Part model, mm, in its own coordinate system. Face numbers are marked on the shaded views. A direction names the side the tool comes from. Round coordinates to 2 decimals unless told otherwise and drop trailing zeros. Write each loop counter-clockwise with the first axis right and the second up, starting at its lowest first coordinate (ties: lowest second). Pieces come first, ordered by that corner, then holes. Notation, with made-up numbers: (-29.75, -17.75) -> (15.25, -17.75) arc R28 ccw to (15.25, 1.25) -> close; hole circle Ø5 at (43, 20.25). An arc over 180 degrees is marked (long way). Use CSV: the item, a comma, the result in double quotes. Start each with the question number.
(1) Saw through at D-D (x = 12). Give the cut face in (y, z), plus the area to 3 significant figures.
(2) Drop flat-ended pins along their axis: pin 1 (1.5 mm diameter, centred on x = -2.5, z = -1, fed in from -Y); pin 2 (1.5 mm diameter, centred on y = 2.5, z = -12, fed in from +X); pin 3 (0.6 mm diameter, centred on x = -3.5, y = 1.5, fed in from +Z). Give the stop position or say it passes through.
(3) Two-plate mould, pull along X, no slides. Class the marked faces 1, 2 and 3: released by +X, released by -X, zero draft, split by the parting line, or undercut.
(4) Saw through at C-C (y = 6.25). Give the cut face in (x, z), plus the area to 3 significant figures.
(5) Saw through at B-B (z = 20). Give the cut face in (x, y), plus the area to 3 significant figures.
(6) Which spindle directions (+Z, -Z, +X, -X, +Y, -Y) get a long thin tool onto all of the face, cutting with end or side? Do the marked faces 4 and 5. Say none if no direction does.
(7) Probe line 1 (Z direction, x = 0, y = 2.7); line 2 (Y direction, x = 5.5, z = -3.5). List the from-to ranges inside material, lowest first. Write a range as [from, to].
(8) Saw through at A-A (x = 0). Give the cut face in (y, z), plus the area to 4 significant figures.
```python
from build123d import *

# Parameters (mm, degrees)
CROQUIS1_R              = 23.5
SALIENTE_EXTRUIR1_DEPTH = 10
CORTAR_EXTRUIR3_DEPTH   = 5
CROQUIS3_R              = 1.25
CORTAR_EXTRUIR4_DEPTH   = 10
CORTAR_EXTRUIR6_DEPTH   = 2


with BuildPart() as part:
    # Croquis1 → Saliente-Extruir1 (new body)
    with BuildSketch(Plane(origin=(0, 0, 0), x_dir=(1, 0, 0), z_dir=(0, 1, 0))):
        Circle(CROQUIS1_R)
    extrude(amount=SALIENTE_EXTRUIR1_DEPTH)

    # Croquis2 → Cortar-Extruir3 (cut)
    with BuildSketch(Plane(origin=(0, 10, 0), x_dir=(1, 0, 0), z_dir=(0, 1, 0))):
        with BuildLine():
            ThreePointArc((3.5, 17), (0, 20.5), (-3.5, 17))
            Line((-3.5, 17), (3.5, 17))
        make_face()
        with BuildLine():
            Line((3.5, 17), (-3.5, 17))
            ThreePointArc((-3.5, 17), (0, 13.5), (3.5, 17))
        make_face()
        with BuildLine():
            Line((-3.5, 6.062177826), (-3.5, 17))
            Line((-3.5, 17), (-6.430705394, 2.765145228))
            ThreePointArc((-6.430705394, 2.765145228), (-5.231857547, 4.650555516), (-3.5, 6.062177826))
        make_face()
        with BuildLine():
            ThreePointArc((3.5, 17), (0, 13.5), (-3.5, 17))
            Line((-3.5, 17), (-3.5, 6.062177826))
            ThreePointArc((-3.5, 6.062177826), (0, 7), (3.5, 6.062177826))
            Line((3.5, 6.062177826), (3.5, 17))
        make_face()
        with BuildLine():
            Line((6.430705394, 2.765145228), (3.5, 17))
            Line((3.5, 17), (3.5, 6.062177826))
            ThreePointArc((3.5, 6.062177826), (5.231857547, 4.650555516), (6.430705394, 2.765145228))
        make_face()
        with BuildLine():
            ThreePointArc((6.430705394, 2.765145228), (5.231857547, 4.650555516), (3.5, 6.062177826))
            Line((3.5, 6.062177826), (3.5, 0))
            Line((3.5, 0), (7, 0))
            Line((7, 0), (6.430705394, 2.765145228))
        make_face()
        with BuildLine():
            ThreePointArc((3.5, 6.062177826), (0, 7), (-3.5, 6.062177826))
            Line((-3.5, 6.062177826), (-3.5, 0))
            Line((-3.5, 0), (3.5, 0))
            Line((3.5, 0), (3.5, 6.062177826))
        make_face()
        with BuildLine():
            Line((3.5, 0), (-3.5, 0))
            Line((-3.5, 0), (-3.5, -6.062177826))
            ThreePointArc((-3.5, -6.062177826), (0, -7), (3.5, -6.062177826))
            Line((3.5, -6.062177826), (3.5, 0))
        make_face()
        with BuildLine():
            ThreePointArc((-3.5, 6.062177826), (-5.231857547, 4.650555516), (-6.430705394, 2.765145228))
            Line((-6.430705394, 2.765145228), (-7, 0))
            Line((-7, 0), (-3.5, 0))
            Line((-3.5, 0), (-3.5, 6.062177826))
        make_face()
        with BuildLine():
            Line((-3.5, 0), (-7, 0))
            ThreePointArc((-7, 0), (-6.062177826, -3.5), (-3.5, -6.062177826))
            Line((-3.5, -6.062177826), (-3.5, 0))
        make_face()
        with BuildLine():
            Line((7, 0), (3.5, 0))
            Line((3.5, 0), (3.5, -6.062177826))
            ThreePointArc((3.5, -6.062177826), (6.062177826, -3.5), (7, 0))
        make_face()
        with BuildLine():
            ThreePointArc((7, 0), (6.856199303, 1.411570445), (6.430705394, 2.765145228))
            Line((6.430705394, 2.765145228), (7, 0))
        make_face()
        with BuildLine():
            Line((-7, 0), (-6.430705394, 2.765145228))
            ThreePointArc((-6.430705394, 2.765145228), (-6.856199303, 1.411570445), (-7, 0))
        make_face()
        with BuildLine():
            ThreePointArc((3.5, -6.062177826), (0, -7), (-3.5, -6.062177826))
            Line((-3.5, -6.062177826), (-3.5, -17))
            Line((-3.5, -17), (3.5, -17))
            Line((3.5, -17), (3.5, -6.062177826))
        make_face()
        with BuildLine():
            ThreePointArc((-3.5, -6.062177826), (-6.062177826, -3.5), (-7, 0))
            Line((-7, 0), (-7, -22.433234274))
            ThreePointArc((-7, -22.433234274), (-3.540409196, -23.231777864), (0, -23.5))
            ThreePointArc((0, -23.5), (3.540409196, -23.231777864), (7, -22.433234274))
            Line((7, -22.433234274), (7, 0))
            ThreePointArc((7, 0), (6.062177826, -3.5), (3.5, -6.062177826))
            Line((3.5, -6.062177826), (3.5, -17))
            Line((3.5, -17), (-3.5, -17))
            Line((-3.5, -17), (-3.5, -6.062177826))
        make_face()
    extrude(amount=-CORTAR_EXTRUIR3_DEPTH, mode=Mode.SUBTRACT)

    # Croquis3 → Cortar-Extruir4 (cut)
    with BuildSketch(Plane(origin=(0, 10, 0), x_dir=(1, 0, 0), z_dir=(0, 1, 0))):
        Circle(CROQUIS3_R)
    extrude(amount=-CORTAR_EXTRUIR4_DEPTH, mode=Mode.SUBTRACT)

    # Croquis5 → Cortar-Extruir6 (cut)
    with BuildSketch(Plane.XZ):
        with BuildLine():
            Line((-7.5, 2.5), (7.5, 2.5))
            ThreePointArc((7.5, 2.5), (10, 0), (7.5, -2.5))
            Line((7.5, -2.5), (-7.5, -2.5))
            ThreePointArc((-7.5, -2.5), (-10, 0), (-7.5, 2.5))
        make_face()
    extrude(amount=-CORTAR_EXTRUIR6_DEPTH, mode=Mode.SUBTRACT)


solid = part.part
```
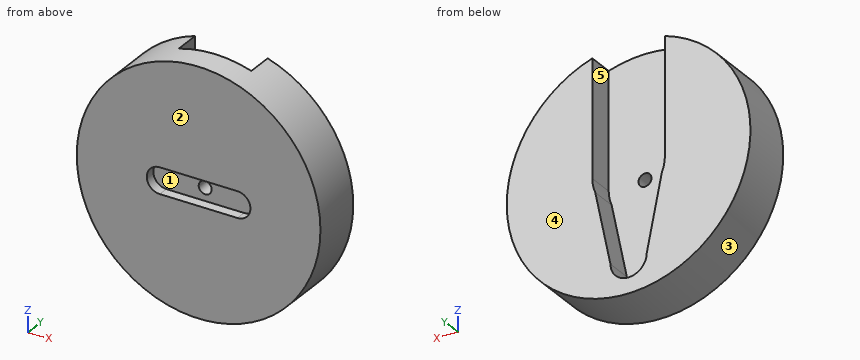
Answers:
1,outline,"(0, -20.21) -> (10, -20.21) -> (10, 20.21) -> (0, 20.21) -> close"
1,area,"404 mm²"
2,pin 1,"stops at y = 2"
2,pin 2,"stops at x = 20.63"
2,pin 3,"stops at z = 23.28"
3,face 1,"undercut"
3,face 2,"zero draft"
3,face 3,"split by the parting line"
4,outline,"(-7, 0) -> (-7, 22.43) arc R23.5 ccw (long way) to (7, 22.43) -> (7, 0) arc R7 cw to (6.43, -2.77) -> (3.5, -17) arc R3.5 cw to (-3.5, -17) -> (-6.43, -2.77) arc R7 cw to start"
4,area,"1,210 mm²"
5,outline,"(-12.34, 0) -> (12.34, 0) -> (12.34, 10) -> (7, 10) -> (7, 5) -> (-7, 5) -> (-7, 10) -> (-12.34, 10) -> close"
5,area,"177 mm²"
6,face 4,"+Z, -Z, +X, -X, +Y"
6,face 5,"+Z, +Y"
7,line 1,"z = [-23.5, -1.25], [1.25, 23.5]"
7,line 2,"y = [0, 5]"
8,outline,"(0, -23.5) -> (10, -23.5) -> (10, -20.5) -> (5, -20.5) -> (5, -1.25) -> (2, -1.25) -> (2, -2.5) -> (0, -2.5) -> close; (0, 2.5) -> (2, 2.5) -> (2, 1.25) -> (5, 1.25) -> (5, 23.5) -> (0, 23.5) -> close"
8,area,"232.5 mm²"
